The figure shows three views and two pictorial views of one solid part (mm, origin at its lowest corner). Answer the questions. A direction names the side the tool comes from. Coordinates: 2 decimals unless noted, no trailing zeros. Loops run counter-clockwise (first coordinate to the right, second up) from the corner with the lowest first, then second, coordinate; pieces in that order, holes last. Notation, with made-up numbers: (86, 22.25) - (144, 22.25) arc R28 cw to (144, 41.25) - close; hole circle Ø1 at (27, 13). An arc over 180 degrees is marked (long way). Write each question's results on one line, items separated by ' | '. Start each with the question number.
Item 1: Consider probe 1 along Y at (x, z) = (27, 1.7); probe 2 along X at (y, z) = (20.5, 12); probe 3 along Y at (x, z) = (27, 2.35). Determine where each line is inside the solid, lowest interval first. Write a range as [from, to].
Item 2: Each of these flat-tipped pins is pushed along its axis until it touches: pin 1 Ø1.5 at (x, z) = (29, 3.5) entering from -Y; pin 2 Ø5.5 at (y, z) = (42.76, 7.5) entering from +X; pin 3 Ø5 at (x, y) = (14.5, 9.5) entering from +Z; pin 4 Ø2.5 at (x, z) = (19, 3.5) entering from +Y. Where does it stop, or does it pass through?
Item 3: Section C-C, the plane x = 15 is taken. Write down the section's boundary in (y, z).
Item 4: Section A-A, the plane y = 22.5 is taken. Write down the section's boundary in (x, z).
Item 5: Section B-B, the plane y = 6 is taken. Write down the section's boundary in (x, z).
Item 6: A tool of negligible diameter and unlimited length cuts with its end or side. For the marked faces 1, 2 and 3, from which of +Z, -Z, +X, -X, +Y, -Y can it reach the whole face along a straight path? Write none if from no direction.
Item 7: Section D-D, the plane z = 6.25 is taken. Write down the section's boundary in (x, y) (1 decimal).
Item 8: For a pull along Y with two mould halves and no side action, classify the marked faces 4, 5 and 6 as +Y half, -Y half, draft (parallel to the pull), parting line (faces both ways), or undercut.
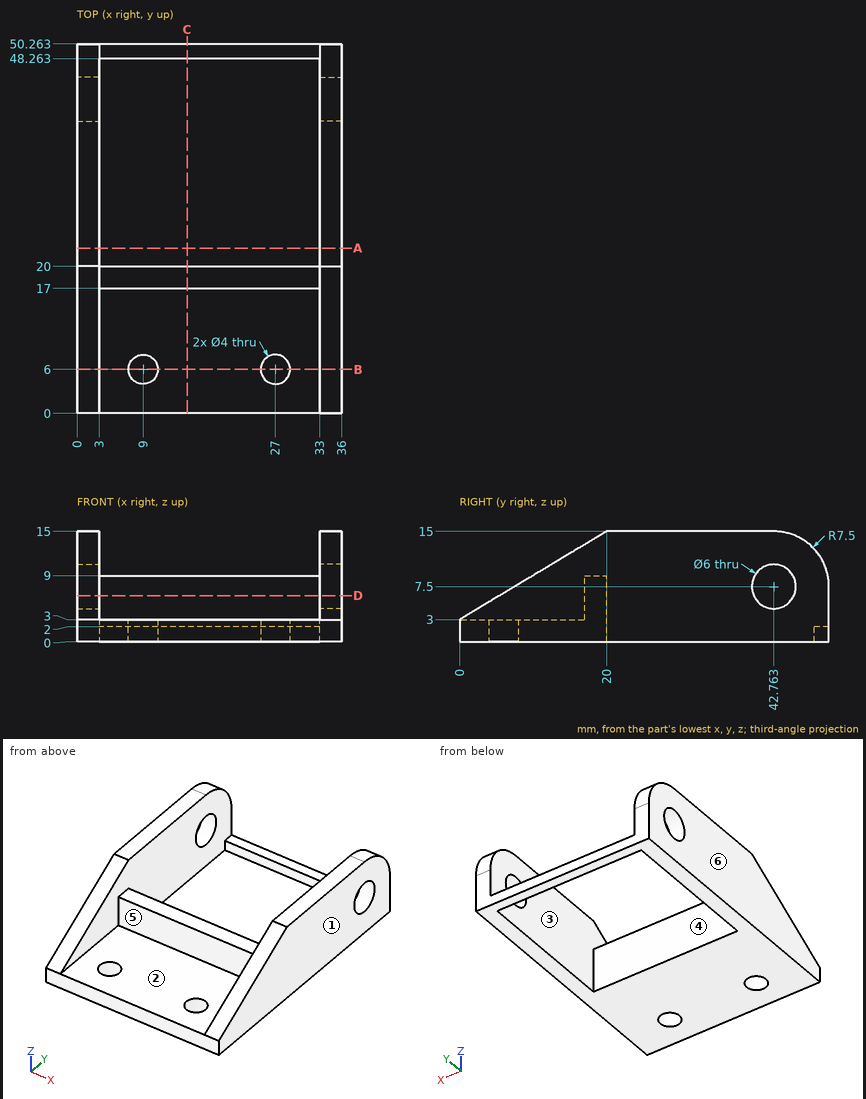
Answer key:
1) probe 1: y = [0, 4], [8, 20], [48.26, 50.26] | probe 2: x = [0, 3], [33, 36] | probe 3: y = [0, 4], [8, 20]
2) pin 1: stops at y = 0 | pin 2: passes through | pin 3: stops at z = 3 | pin 4: stops at y = 20
3) outline: (0, 0) - (20, 0) - (20, 9) - (17, 9) - (17, 3) - (0, 3) - close; (48.26, 0) - (50.26, 0) - (50.26, 2) - (48.26, 2) - close
4) outline: (0, 0) - (3, 0) - (3, 15) - (0, 15) - close; (33, 0) - (36, 0) - (36, 15) - (33, 15) - close
5) outline: (0, 0) - (7, 0) - (7, 3) - (3, 3) - (3, 6.6) - (0, 6.6) - close; (11, 0) - (25, 0) - (25, 3) - (11, 3) - close; (29, 0) - (36, 0) - (36, 6.6) - (33, 6.6) - (33, 3) - (29, 3) - close
6) face 1: +Z, -Z, +X, +Y, -Y | face 2: +Z, -Y | face 3: +Z
7) outline: (0, 5.4) - (3, 5.4) - (3, 17) - (33, 17) - (33, 5.4) - (36, 5.4) - (36, 40) - (33, 40) - (33, 20) - (3, 20) - (3, 40) - (0, 40) - close; (0, 45.5) - (3, 45.5) - (3, 50.3) - (0, 50.3) - close; (33, 45.5) - (36, 45.5) - (36, 50.3) - (33, 50.3) - close
8) face 4: undercut | face 5: -Y half | face 6: draft
